The listing builds one solid part. Answer for the finished solid, in the listing's coordinates (mm). Face numbers are marked on the shaded views. A direction names the side the tool comes from. Give positions to 0.01 mm unless a question says otherwise; leave off trailing zeros. Order: outer loops, then holes, each group sorted by start corner. A loop starts at its lowest first (then second) coordinate and runs counter-clockwise, first axis right, second up. Notation, with made-up numbers: (65.25, -14) - (71.25, -14) arc R38 ccw to (71.25, 25) - close; hole circle Ø8 at (15, -32.75). An arc over 180 degrees is marked (long way). Answer as CSV lines item,"result". Start each with the question number.
1. Which of the six approach directions +Z, -Z, +X, -X, +Y, -Y give full straight-line access (tool end or side, diameter ignored) to the marked faces 4 and 5?
2. Section B-B on z = 10.25 is taken. Give the vertices of the cut face in (x, y).
3. Section D-D on z = 7.5 is taken. Give the vertices of the cut face in (x, y).
4. Consider line 1 along Y through (x, z) = (0, 3.25); line 2 along X through (y, z) = (0, 5.5); line 3 along X through (y, z) = (2.5, 10.5). Determine where each line is inside the solid, lowest interval first. Write a range as [from, to].
5. Section A-A on y = 0 is taken. Give the vertices of the cut face in (x, z).
6. Flat-ended cylindrical pins translate along their axes: pin 1 (1.5 mm diameter, centred on y = -1, z = 4, fed in from -X); pin 2 (4 mm diameter, centred on x = 0.5, y = 0, fed in from +Z); pin 3 (2.5 mm diameter, centred on y = 0, z = 13, fed in from -X). Find the tip coordinate at first contact, or state that the pin passes through.
7. Section C-C on x = -3.25 is taken. Give the vertices of the cut face in (y, z), and give its area (3 significant figures).
8. Determine the mould class of the marked faces 1, 2 and 3 for opening direction X: +X half, -X half, draft (parallel to the pull), parting line (faces both ways), or undercut.
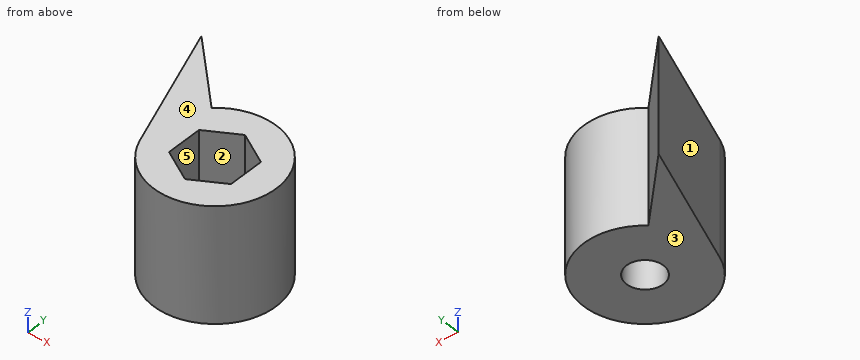
from build123d import *

# Parameters (mm, degrees)
CLONE027_ROLL_ANGLE = 90
PAD014_DEPTH        = 10
PAD006_DEPTH        = 15


with BuildPart() as clone_of_m5countersinkslot002:
    # Sketch013 → Revolution (revolve)
    with BuildSketch(Plane.XY):
        Polygon((0, 20), (5, 20), (5, 0), (2.4, -2.6), (2.4, -45), (0, -45), align=None)
    revolve(axis=Axis((0, 0, 0), (0, 1, 0)))


with BuildPart() as clone_of_m5countersinkslot002_1:
    # Clone027 roll: moved
    add(clone_of_m5countersinkslot002.part.rotate(Axis((0, 0, 0), (1, 0, 0)), CLONE027_ROLL_ANGLE))


with BuildPart() as clone_of_m5countersinkslot002_2:
    # Clone027 placement: moved
    add(clone_of_m5countersinkslot002_1.part.moved(Location((0, 0, 26))))


with BuildPart() as clone_of_din934slot001:
    # Sketch014 → Pad014 (new body)
    with BuildSketch(Plane.XY):
        Polygon((4.05, -2.338269), (4.05, 2.338269), (0, 4.676537), (-4.05, 2.338269), (-4.05, -2.338269), (0, -4.676537), align=None)
    extrude(amount=PAD014_DEPTH)


with BuildPart() as clone_of_din934slot001_1:
    # Clone026 placement: moved
    add(clone_of_din934slot001.part.moved(Location((0, 0, 8))))


with BuildPart() as normalhinge:
    # Clone2D001 → Pad006 (new body)
    with BuildSketch(Plane.XY):
        with BuildLine():
            ThreePointArc((-7.517553, -2.736129), (7.769812, -1.90526), (-5.399017, 5.903441))
            Line((-5.399017, 5.903441), (-13.673915, 14.178338))
            Line((-13.673915, 14.178338), (-7.517553, -2.736129))
        make_face()
    extrude(amount=PAD006_DEPTH)

    # Cut017: cut Clone of DIN934Slot001
    add(clone_of_din934slot001_1.part, mode=Mode.SUBTRACT)

    # Cut007: cut Clone of M5CounterSinkSlot002
    add(clone_of_m5countersinkslot002_2.part, mode=Mode.SUBTRACT)


solid = normalhinge.part
Checks:
1,face 4,"+Z, +X, -X, +Y, -Y"
1,face 5,"+Z"
2,outline,"(-13.67, 14.18) - (-7.52, -2.74) arc R8 ccw (long way) to (-5.4, 5.9) - close; hole (-4.05, -2.34) - (0, -4.68) - (4.05, -2.34) - (4.05, 2.34) - (0, 4.68) - (-4.05, 2.34) - close"
3,outline,"(-13.67, 14.18) - (-7.52, -2.74) arc R8 ccw (long way) to (-5.4, 5.9) - close; hole circle Ø4.8 at (0, 0)"
4,line 1,"y = [-8, -2.4], [2.4, 8]"
4,line 2,"x = [-8.51, -2.4], [2.4, 8]"
4,line 3,"x = [-9.42, -3.77], [3.77, 7.6]"
5,outline,"(-8.51, 0) - (-2.4, 0) - (-2.4, 8) - (-4.05, 8) - (-4.05, 15) - (-8.51, 15) - close; (2.4, 0) - (8, 0) - (8, 15) - (4.05, 15) - (4.05, 8) - (2.4, 8) - close"
6,pin 1,"stops at x = -8.42"
6,pin 2,"stops at z = 8"
6,pin 3,"stops at x = -8.97"
7,outline,"(-7.31, 0) - (7.31, 0) - (7.31, 15) - (2.8, 15) - (2.8, 8) - (-2.8, 8) - (-2.8, 15) - (-7.31, 15) - close"
7,area,"180 mm²"
8,face 1,"-X half"
8,face 2,"undercut"
8,face 3,"draft"
